Source: CAD feature listing. Evaluate the final solid. Frame: model axes, mm. A direction names the side the tool comes from. Coordinates: 2 decimals unless noted, no trailing zeros. Loops run counter-clockwise (first coordinate to the right, second up) from the corner with the lowest first, then second, coordinate; pieces in that order, holes last. Notation, with made-up numbers: (-2, -34) - (32, -34) arc R18 ccw to (32, -25) - close; hole circle Ø10 at (1.5, -1.5). An arc over 180 degrees is marked (long way). Use CSV: the item, a comma, the result in double quotes. Start each with the question number.
```python
from build123d import *

# Parameters (mm, degrees)
SZKIC1_W                        = 27
SZKIC1_H                        = 25
ZAOKR_GLENIE1_R                 = 4
SZKIC4_R                        = 3
WYTNIJ_WYCI_GNI_CIE3_DEPTH      = 24.0000001
WYTNIJ_WYCI_GNI_CIE3_DEPTH_BACK = 3
WYTNIJ_WYCI_GNI_CIE2_DEPTH      = 24.0000001
SZKIC5_OUTSIDE_W                = 72.072
SZKIC5_OUTSIDE_H                = 72.072
WYTNIJ_WYCI_GNI_CIE4_DEPTH      = 26.0000001
SZKIC8_W                        = 8.35
SZKIC8_H                        = 12
SZKIC10_R                       = 3.5
WYTNIJ_WYCI_GNI_CIE5_DEPTH      = 56.423393859


with BuildPart() as part:
    # Szkic1 → Obrót1 (revolve)
    with BuildSketch(Plane.XY):
        with Locations((13.5, 12.5)):
            Rectangle(SZKIC1_W, SZKIC1_H)
    revolve(axis=Axis((0, 0, 0), (0, 1, 0)))

    # Szkic2 → Wycięcie-obrót1 (revolve, cut)
    with BuildSketch(Plane.XY):
        Polygon((27, 25), (27, 2), (8.35, 8.788044869), (8.35, 25), align=None)
    revolve(axis=Axis((0, 0, 0), (0, 1, 0)), mode=Mode.SUBTRACT)

    # Zaokrąglenie1
    zaokr_glenie1_edges = [part.edges().sort_by_distance(p)[0] for p in [
        (-8.35, 8.788044869, 0),
    ]]
    fillet(zaokr_glenie1_edges, radius=ZAOKR_GLENIE1_R)

    # Szkic4 → Wytnij-wyciągnięcie3 (cut, two sides)
    with BuildSketch(Plane(origin=(0, 2, 0), x_dir=(1, 0, 0), z_dir=(0, 1, 0))) as wytnij_wyci_gni_cie3_sk:
        with Locations((-20, 0)):
            Circle(SZKIC4_R)
        with Locations((20, 0)):
            Circle(SZKIC4_R)
    extrude(amount=WYTNIJ_WYCI_GNI_CIE3_DEPTH, mode=Mode.SUBTRACT)
    extrude(wytnij_wyci_gni_cie3_sk.sketch, amount=-WYTNIJ_WYCI_GNI_CIE3_DEPTH_BACK, mode=Mode.SUBTRACT)

    # Szkic3 → Wytnij-wyciągnięcie2 (cut, through all)
    with BuildSketch(Plane(origin=(0, 2, 0), x_dir=(1, 0, 0), z_dir=(0, 1, 0))):
        with BuildLine():
            Line((-17.5, 5), (-26.532998323, 5))
            ThreePointArc((-26.532998323, 5), (-27, 0), (-26.532998323, -5))
            Line((-26.532998323, -5), (-17.5, -5))
            ThreePointArc((-17.5, -5), (-12.5, 0), (-17.5, 5))
        make_face()
        with BuildLine():
            Line((17.5, 5), (26.532998323, 5))
            ThreePointArc((26.532998323, 5), (27, 0), (26.532998323, -5))
            Line((26.532998323, -5), (17.5, -5))
            ThreePointArc((17.5, -5), (12.5, 0), (17.5, 5))
        make_face()
    extrude(amount=WYTNIJ_WYCI_GNI_CIE2_DEPTH, mode=Mode.SUBTRACT)

    # Szkic5 outside → Wytnij-wyciągnięcie4 (cut, through all)
    with BuildSketch(Plane.XZ):
        Rectangle(SZKIC5_OUTSIDE_W, SZKIC5_OUTSIDE_H)
        with BuildLine():
            Line((-20.2625, 6.995076393), (-0.290625, 7.744548864))
            ThreePointArc((-0.290625, 7.744548864), (0, 7.75), (0.290625, 7.744548864))
            Line((0.290625, 7.744548864), (20.2625, 6.995076393))
            ThreePointArc((20.2625, 6.995076393), (27, 0), (20.2625, -6.995076393))
            Line((20.2625, -6.995076393), (0.290625, -7.744548864))
            ThreePointArc((0.290625, -7.744548864), (0, -7.75), (-0.290625, -7.744548864))
            Line((-0.290625, -7.744548864), (-20.2625, -6.995076393))
            ThreePointArc((-20.2625, -6.995076393), (-27, 0), (-20.2625, 6.995076393))
        make_face(mode=Mode.SUBTRACT)
    extrude(amount=-WYTNIJ_WYCI_GNI_CIE4_DEPTH, mode=Mode.SUBTRACT)

    # Szkic8 → Wycięcie-obrót2 (revolve, cut)
    with BuildSketch(Plane.XY):
        with Locations((4.175, 19)):
            Rectangle(SZKIC8_W, SZKIC8_H)
    revolve(axis=Axis((0, 25, 0), (0, -1, 0)), mode=Mode.SUBTRACT)

    # Szkic9 → Obrót2 (revolve)
    with BuildSketch(Plane.XY):
        Polygon((6, 55.423393759), (0, 55.423393759), (0, 13), (6.95, 13), (6.95, 52.423393759), (7, 52.423393759), (7, 54.423393759), align=None)
    revolve(axis=Axis((0, 13, 0), (0, 1, 0)))

    # Szkic10 → Wytnij-wyciągnięcie5 (cut, through all)
    with BuildSketch(Plane(origin=(0, 55.423393759, 0), x_dir=(1, 0, 0), z_dir=(0, 1, 0))):
        Circle(SZKIC10_R)
    extrude(amount=-WYTNIJ_WYCI_GNI_CIE5_DEPTH, mode=Mode.SUBTRACT)


solid = part.part
```
(1) Pin query (flat end, axial travel): pin 1 Ø1 at (x, z) = (21, -3.5) entering from +Y; pin 2 Ø6 at (x, y) = (20, 8.5) entering from -Z; pin 3 Ø3.5 at (x, y) = (20.5, 3) entering from +Z; pin 4 Ø3.5 at (x, y) = (-21.5, 4) entering from +Z. Return the tip coordinate at first contact, or that it passes through.
(2) Ray query, line 1 (Z direction, x = 20, y = 0.9); line 2 (X direction, y = 51, z = -0.25); line 3 (Z direction, x = 0, y = 43). Return the intervals inside material, ascending. Write a range as [from, to].
(3) Section B-B on z = 1.75. State how many separate pieces and enclosed holes the cut face has, plus the area to 3 significant figures.
(4) Draft query along Z for faces 1 (the flat face through (3, 55.423, 3)), 2 (the cylindrical face through (-27, 1.54, -0.15)), 3 (the cylindrical face through (17, 1, 0)). Return one class per face: released by +Z, released by -Z, zero draft, split by the parting line, or undercut.
(5) Section A-A on y = 30. Output: boundary loops of the cut face in (x, z).
(6) Reachability of faces 4 (the flat face through (23, 2, -1)), 5 (the cylindrical face through (-1.507, 32.988, 6.785)), 6 (the flat face through (-20, 3, 5)) from +Z, -Z, +X, -X, +Y, -Y: full face, straight path, thin tool, end or side. Return the list, or none.
Solution:
1,pin 1,"stops at y = 2"
1,pin 2,"passes through"
1,pin 3,"stops at z = 7.05"
1,pin 4,"stops at z = 7.01"
2,line 1,"z = [-7, -3], [3, 7]"
2,line 2,"x = [-6.95, -3.49], [3.49, 6.95]"
2,line 3,"z = [-6.95, -3.5], [3.5, 6.95]"
3,separate pieces,"4"
3,enclosed holes,"0"
3,area,"560 mm²"
4,face 1,"zero draft"
4,face 2,"split by the parting line"
4,face 3,"undercut"
5,outline,"circle Ø13.9 at (0, 0); hole circle Ø7 at (0, 0)"
6,face 4,"+X, +Y"
6,face 5,"none"
6,face 6,"-X, +Y"
